from build123d import *

# Parameters (mm, degrees)
F0_R     = 35.231232
F1_DEPTH = 127
F2_W     = 17.652087
F2_H     = 57.944892


with BuildPart() as f1:
    # F0 (on Top) → F1 (new body)
    with BuildSketch(Plane.XY):
        Circle(F0_R)
    extrude(amount=F1_DEPTH)

    # F2 (on Right) → F4 (revolve, cut)
    with BuildSketch(Plane.YZ):
        with Locations((-26.47813, 57.442375)):
            Rectangle(F2_W, F2_H)
    revolve(axis=Axis((0, 0, 50.498489), (0, 0, 1)), mode=Mode.SUBTRACT)


solid = f1.part
Design review of the part built by this model. Coordinates are the model's own, in mm. A direction names the side the tool comes from. Give positions to 0.01 mm unless a question says otherwise; leave off trailing zeros. Write each loop counter-clockwise with the first axis right and the second up, starting at its lowest first coordinate (ties: lowest second). Pieces come first, ordered by that corner, then holes. Notation, with made-up numbers: M 44.5,60.25 L 57.5,60.25 A8 cw 57.5,73.25 Z; hole C 88.5,71 d3. An arc over 180 degrees is marked long. Return JSON: item names as keys, results as strings. Group by question number.
Item 1: Take a section at D-D (z = 62.5). Give the boundary of the cut face in (x, y).
Item 2: Take a section at A-A (x = -30). Give the boundary of the cut face in (y, z).
Item 3: Tool access review of faces 1 (the flat face through (0, 0, 127)), 2 (the cylindrical face through (5.302, -16.837, 57.848)): name each direction out of +Z, -Z, +X, -X, +Y, -Y from which nothing blocks a thin tool from reaching the whole face with its end or side.
Item 4: Clearance check with flat-ended pins moving along their axes: pin 1 Ø5 at (y, z) = (-3.5, 88) entering from -X; pin 2 Ø6 at (y, z) = (23, 17) entering from -X; pin 3 Ø4 at (y, z) = (11, 78.5) entering from -X. State where each tip first meets the part, or that it passes through.
Item 5: Take a section at C-C (x = 0). Give the boundary of the cut face in (y, z).
Item 6: Wall thickness on line 1 along Z through (x, y) = (27, -21); line 2 along X through (y, z) = (0.5, 107); line 3 along Y through (x, z) = (6, 16): over which ranges is each line inside the solid? List them lowest first.
Item 7: Take a section at B-B (y = -28). Give the boundary of the cut face in (x, z).
Item 8: The part is to be moulded in two halves that separate along Z. For faces 3 (the flat face through (8, 16, 28.47)), 4 (the flat face through (0, 0, 0)), 5 (the cylindrical face through (-4.59, 34.93, 106.42)), say which applies: pulls with the +Z half, pulls with the -Z half, needs draft (parallel to the pull), parting line crosses it, or undercut.
Return value:
{
 "1": {"outline": "C 0,0 d35.3"},
 "2": {"outline": "M -18.47,0 L 18.47,0 L 18.47,28.47 L -18.47,28.47 Z; M -18.47,86.41 L 18.47,86.41 L 18.47,127 L -18.47,127 Z"},
 "3": {"face 1": "+Z, +X, -X, +Y, -Y", "face 2": "none"},
 "4": {"pin 1": "stops at x = -35.22", "pin 2": "stops at x = -29", "pin 3": "stops at x = -15.19"},
 "5": {"outline": "M -35.23,0 L 35.23,0 L 35.23,28.47 L 17.65,28.47 L 17.65,86.41 L 35.23,86.41 L 35.23,127 L -35.23,127 L -35.23,86.41 L -17.65,86.41 L -17.65,28.47 L -35.23,28.47 Z"},
 "6": {"line 1": "z = 0 to 28.47, 86.41 to 127", "line 2": "x = -35.23 to 35.23", "line 3": "y = -34.72 to 34.72"},
 "7": {"outline": "M -21.38,0 L 21.38,0 L 21.38,28.47 L -21.38,28.47 Z; M -21.38,86.41 L 21.38,86.41 L 21.38,127 L -21.38,127 Z"},
 "8": {"face 3": "undercut", "face 4": "pulls with the -Z half", "face 5": "needs draft"}
}
